The listing builds one solid part. Answer for the finished solid, in the listing's coordinates (mm). A direction names the side the tool comes from. Coordinates: 2 decimals unless noted, no trailing zeros. Order: outer loops, then holes, each group sorted by start corner. A loop starts at its lowest first (then second) coordinate and runs counter-clockwise, first axis right, second up. Notation, with made-up numbers: (-22.75, 49.5) -> (-8.75, 49.5) arc R17 cw to (-8.75, 68.5) -> close; hole circle Ø11 at (26.5, 77.25). An arc over 180 degrees is marked (long way). Return JSON: item names as keys, results as strings.
from build123d import *

# Parameters (mm, degrees)
F3_DEPTH      = 5
F3_DEPTH_BACK = 5
F5_COUNT      = 6
F6_R          = 30
F6_R_2        = 15
F8_DEPTH      = 8.3061646
F8_DEPTH_BACK = 8.3061646


# Not quite as in the source:
# - an extrude ends at something that could not be found from the text; its depth is read off the source's solid
# - a feature of the source that left no trace in its solid (it failed there, or was rolled back) is left out


with BuildPart() as f3:
    # F2 (on line) → F3 (new body, two sides)
    with BuildSketch(Plane(origin=(0, 0, 0), x_dir=(1, 0, 0), z_dir=(0, 0.5, -0.8660254038))) as f3_sk:
        with BuildLine():
            ThreePointArc((25, 0), (24.7861215343, -3.2631548055), (24.1481456572, -6.4704761276))
            Line((24.1481456572, -6.4704761276), (96.5925826289, -25.8819045103))
            ThreePointArc((96.5925826289, -25.8819045103), (99.1444861374, -13.052619222), (100, 0))
            ThreePointArc((100, 0), (99.1444861374, 13.052619222), (96.5925826289, 25.8819045103))
            Line((96.5925826289, 25.8819045103), (24.1481456572, 6.4704761276))
            ThreePointArc((24.1481456572, 6.4704761276), (24.7861215343, 3.2631548055), (25, 0))
        make_face()
    extrude(amount=F3_DEPTH)
    extrude(f3_sk.sketch, amount=-F3_DEPTH_BACK)


with BuildPart() as f5_1:
    # F5: instance of F3
    add(f3.part.rotate(Axis((0, 0, -4.0518213063), (0, 0, -1)), 1 * 360 / F5_COUNT))


with BuildPart() as f5_2:
    # F5: instance of F3
    add(f3.part.rotate(Axis((0, 0, -4.0518213063), (0, 0, -1)), 2 * 360 / F5_COUNT))


with BuildPart() as f5_3:
    # F5: instance of F3
    add(f3.part.rotate(Axis((0, 0, -4.0518213063), (0, 0, -1)), 3 * 360 / F5_COUNT))


with BuildPart() as f5_4:
    # F5: instance of F3
    add(f3.part.rotate(Axis((0, 0, -4.0518213063), (0, 0, -1)), 4 * 360 / F5_COUNT))


with BuildPart() as f5_5:
    # F5: instance of F3
    add(f3.part.rotate(Axis((0, 0, -4.0518213063), (0, 0, -1)), 5 * 360 / F5_COUNT))


with BuildPart() as f3_1:
    add(f3.part)

    add(f5_1.part)  # F8 merges F5_1

    add(f5_2.part)  # F8 merges F5_2

    add(f5_3.part)  # F8 merges F5_3

    add(f5_4.part)  # F8 merges F5_4

    add(f5_5.part)  # F8 merges F5_5
    # F6 (on Top) → F8 (join, two sides)
    with BuildSketch(Plane.XY) as f8_sk:
        Circle(F6_R)
        Circle(F6_R_2, mode=Mode.SUBTRACT)
    extrude(amount=F8_DEPTH)
    extrude(f8_sk.sketch, amount=-F8_DEPTH_BACK)


solid = f3_1.part
1. For faces 1 (the face through (43.566, -46.564, 8.26)), 2 (the face through (-44.17, -47.31, -8.51)), 3 (the face through (0, 30, 0)), 4 (the face through (-18.54, -61.01, 8.26)), determine the directions among +Z, -Z, +X, -X, +Y, -Y from which every point of the face is accessible in a straight line to the end or side of a thin tool.
Answer block:
{"face 1": "+Z, +X", "face 2": "-Z, -X", "face 3": "+Y", "face 4": "+Z, -Y"}
2. Consider line 1 (Y direction, x = 0, z = 1.5); line 2 (X direction, y = -65.5, z = -8); line 3 (X direction, y = 57.5, z = 8.5). Determine where each line is inside the solid, lowest interval first. Write a range as from..to.
Answer block:
{"line 1": "y = -30..-15, 15..30", "line 2": "x = -64.22..-42.27, 19.42..33.36", "line 3": "x = -55.18..-38.65, 17.88..27.74"}
3. The part is cut by section C-C on x = -73.5. Give the vertices of the cut face in (y, z).
Answer block:
{"outline": "(-19.56, 5.52) -> (14.56, -14.18) -> (19.56, -5.52) -> (-14.56, 14.18) -> close"}
4. The part is cut by section B-B on y = -68. Give the vertices of the cut face in (x, z), and give its area (3 significant figures).
Answer block:
{"outline": "(-66.89, -8.04) -> (-60.22, -16.25) -> (-18.16, 4.78) -> (-23.25, 13.78) -> close; (18.16, -4.78) -> (23.25, -13.78) -> (66.89, 8.04) -> (60.22, 16.25) -> close", "area": "990 mm2"}
5. The part is cut by section A-A on x = 0. Give the vertices of the cut face in (y, z).
Answer block:
{"outline": "(-30, -8.31) -> (-15, -8.31) -> (-15, 8.31) -> (-30, 8.31) -> close; (15, -8.31) -> (30, -8.31) -> (30, 8.31) -> (15, 8.31) -> close"}
6. Each of these flat-tipped pins is pushed along its axis until it touches: pin 1 Ø18 at (x, y) = (11, -15) entering from -Z; pin 2 Ø5 at (y, z) = (42, -4.5) entering from +X; pin 3 Ø3 at (x, z) = (-76, -2) entering from -Y. Where does it stop, or does it pass through?
Answer block:
{"pin 1": "stops at z = -8.31", "pin 2": "stops at x = 44.84", "pin 3": "stops at y = -9.13"}
7. The part is cut by section D-D on x = -33.5. Give the number of separate pieces and of enclosed holes in the cut face, and give its area (3 significant figures).
Answer block:
{"separate pieces": "3", "enclosed holes": "0", "area": "1,510 mm2"}
8. Determine the mould class of faces 5 (the face through (-33.43, 63.52, 4.15)), 6 (the face through (-49.69, -86.78, 0.12)), 7 (the face through (-71.72, 2.81, 4.15)) for opening direction X: pulls with the +X half, pulls with the -X half, needs draft (parallel to the pull), parting line crosses it, or undercut.
Answer block:
{"face 5": "undercut", "face 6": "pulls with the -X half", "face 7": "needs draft"}
